Autodesk Inventor part; units mm, degrees
ref_plane "YZ Plane" through (0, 0, 0) normal (1, 0, 0) x (0, 1, 0)
ref_plane "XZ Plane" through (0, 0, 0) normal (0, 1, 0) x (-1, 0, 0)
ref_plane "XY Plane" through (0, 0, 0) normal (0, 0, 1) x (1, 0, 0)
sketch "Эскиз1" plane through (0, 0, 0) normal (0, 1, 0) x (-1, 0, 0)
  circle A0 centre (0, 0) radius 90
  dimension "d0" = 180
extrude "Выдавливание1" add sketch "Эскиз1" along normal blind 8
sketch "Эскиз2" plane through (0, 8, 0) normal (0, 1, 0) x (1, 0, 0)
  circle A0 centre (0, 0) radius 70
  dimension "d3" = 140
extrude "Выдавливание2" add sketch "Эскиз2" along normal blind 65
hole "Отверстие1" at (-1.069, 73, 0) direction (0, -1, 0) diameter 115 depth 10 tip angle 118
hole "Отверстие2" at (-0.208, 0, -0.4159) direction (0, 1, 0) diameter 130 depth 63 tip angle 118
chamfer "Фаска1" distance 2 angle 45 1 edges at (-70, 73, 0)
chamfer "Фаска2" distance 1 angle 45 1 edges at (-0.208, 0, 64.5841)
sketch "Эскиз3" plane through (0, 8, 0) normal (0, 1, 0) x (1, 0, 0)
  circle A0 centre (0, 0) radius 80
  circle A1 centre (80, 0) radius 5.5
  circle A2 centre (40, -69.282) radius 5.5
  circle A3 centre (-40, -69.282) radius 5.5
  circle A4 centre (-80, 0) radius 5.5
  circle A5 centre (-40, 69.282) radius 5.5
  circle A6 centre (40, 69.282) radius 5.5
  dimension "d30" = 160
  dimension "d31" = 11
  dimension "d34" = 360
extrude "Выдавливание3" cut sketch "Эскиз3" against normal blind 100 contours A0 A1 | A0 A1 | A6 A0 | A0 A6 | A2 A0 | A0 A2 | A5 A0 | A0 A5 | A3 A0 | A0 A3 | A4 A0 | A0 A4
sketch "Эскиз4" plane through (0, 0, 0) normal (0, -1, 0) x (1, 0, 0)
  point P0 (0, 0)
Geometry check sheet. Reference: the model listing, model coordinates, mm. A direction names the side the tool comes from. Round coordinates to 2 decimals unless told otherwise and drop trailing zeros. Order: outer loops, then holes, each group sorted by start corner. A loop starts at its lowest first (then second) coordinate and runs counter-clockwise, first axis right, second up. Notation, with made-up numbers: M -39,87 L 14,87 A30 cw 14,117 Z; hole C 0.5,63.5 d5. An arc over 180 degrees is marked long. Answer in a Markdown table with one row per item. Add a question column.
Item 1: Set-up check for faces 5 (the face through (-46, 8, -53)), 6 (the face through (34.505, 4.056, 69.04)), 7 (the face through (-19.732, 32.434, -62.414)): record each of +Z, -Z, +X, -X, +Y, -Y from which the full face is reachable in a straight line by a thin tool's end or side.
Item 2: Material ranges on L1, parallel to X at y = 4.5, z = 71.5; L2, parallel to Z at x = 40, y = 5.5; L3, parallel to X at y = 17.5, z = -4.5, recorded low to high. Write a range as [from, to].
Item 3: Sectioned sample at B-B, the plane x = -40. State how many separate pieces and enclosed holes the cut face has, plus the area to 3 significant figures.
Item 4: Depth check by flat-ended pin: pin 1 Ø6 at (x, z) = (-66.5, -49.5) entering from +Y; pin 2 Ø12.5 at (x, z) = (-40, -69.282) entering from -Y; pin 3 Ø10 at (x, z) = (40, 69.282) entering from +Y; pin 4 Ø6 at (x, y) = (-9.5, 55.5) entering from +Z. Enter the tip coordinate at first touch or a pass-through.
Item 5: Draft check along X on faces 1 (the face through (74.505, 4.056, -0.242)), 2 (the face through (-55.55, 39.059, -42.594)), 3 (the face through (45, 73, 35)), 4 (the face through (-49.553, 69.923, 30.912)). Enter one of: released by +X, released by -X, zero draft, split by the parting line, or undercut.
Item 6: Sectioned sample at D-D, the plane y = 22.5. Enter the section's corners in (x, z).
Item 7: Sectioned sample at A-A, the plane x = 80. Enter the section's corners in (y, z), plus the area to 3 significant figures.
Filled in:
| question | item | result |
|---|---|---|
| 1 | face 5 | +Y |
| 1 | face 6 | +Y, -Y |
| 1 | face 7 | -Y |
| 2 | L1 | x = [-54.66, -45.03], [-34.97, 34.97], [45.03, 54.66] |
| 2 | L2 | z = [-80.62, -74.78], [-63.78, -51.49], [50.66, 63.78], [74.78, 80.62] |
| 2 | L3 | x = [-69.86, -65.08], [64.66, 69.86] |
| 3 | separate pieces | 4 |
| 3 | enclosed holes | 0 |
| 3 | area | 1,220 mm² |
| 4 | pin 1 | stops at y = 8 |
| 4 | pin 2 | stops at y = 0 |
| 4 | pin 3 | passes through |
| 4 | pin 4 | stops at z = 69.7 |
| 5 | face 1 | undercut |
| 5 | face 2 | split by the parting line |
| 5 | face 3 | zero draft |
| 5 | face 4 | undercut |
| 6 | outline | C 0,0 d140; hole C -0.21,-0.42 d130 |
| 7 | outline | M 0,-41.23 L 8,-41.23 L 8,-5.5 L 0,-5.5 Z; M 0,5.5 L 8,5.5 L 8,41.23 L 0,41.23 Z |
| 7 | area | 572 mm² |
